Geometry check sheet. Reference: drawing and pictorial views, mm from the part's lowest x, y, z. Coordinates: 2 decimals unless noted, no trailing zeros. Loops run counter-clockwise (first coordinate to the right, second up) from the corner with the lowest first, then second, coordinate; pieces in that order, holes last.
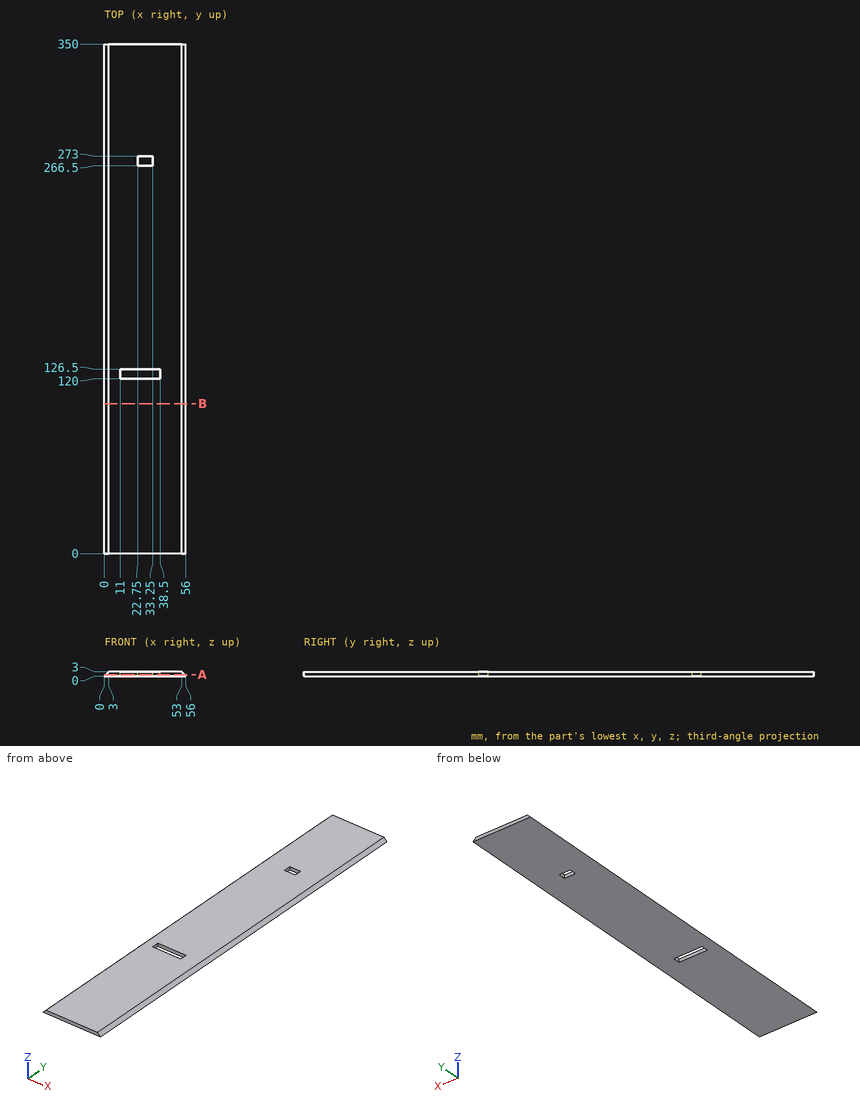
1) Section check B-B on y = 103. Record the cut outline in (x, z), and give its area (3 significant figures).
Data:
outline: (0, 0) - (56, 0) - (53, 3) - (3, 3) - close
area: 159 mm2
2) Material ranges on probe 1 along Y at (x, z) = (35, 1.9); probe 2 along Y at (x, z) = (23, 1.4); probe 3 along X at (y, z) = (284.5, 2.95), recorded low to high.
Data:
probe 1: y = 0 to 120, 126.5 to 350
probe 2: y = 0 to 120, 126.5 to 266.5, 273 to 350
probe 3: x = 2.95 to 53.05
3) Depth check by flat-ended pin: pin 1 (1.5 mm diameter, centred on y = 269, z = 2, fed in from +X); pin 2 (1 mm diameter, centred on x = 34.5, z = 0.5, fed in from -Y); pin 3 (1.5 mm diameter, centred on y = 270, z = 2, fed in from -X); pin 4 (1.5 mm diameter, centred on y = 122, z = 1.5, fed in from -X). Enter the tip coordinate at first touch or a pass-through.
Data:
pin 1: stops at x = 54.75
pin 2: stops at y = 0
pin 3: stops at x = 1.25
pin 4: stops at x = 0.75
4) Section check A-A on z = 0.9. Record the cut outline in (x, y).
Data:
outline: (0.9, 0) - (55.1, 0) - (55.1, 350) - (0.9, 350) - close; hole (11, 120) - (38.5, 120) - (38.5, 126.5) - (11, 126.5) - close; hole (22.75, 266.5) - (33.25, 266.5) - (33.25, 273) - (22.75, 273) - close
